Check sheet for the modelled part. Datum: model origin and axes. Units: mm. Face numbers are marked on the shaded views. A direction names the side the tool comes from. Give positions to 0.01 mm unless a question says otherwise; leave off trailing zeros. Loops run counter-clockwise (first coordinate to the right, second up) from the corner with the lowest first, then second, coordinate; pieces in that order, holes last. Notation, with made-up numbers: M 12,63.5 L 33,63.5 A19 ccw 33,93.5 Z; hole C 32.5,76 d7. An arc over 180 degrees is marked long. Put each result on its own line as item: value. Start each with the question number.
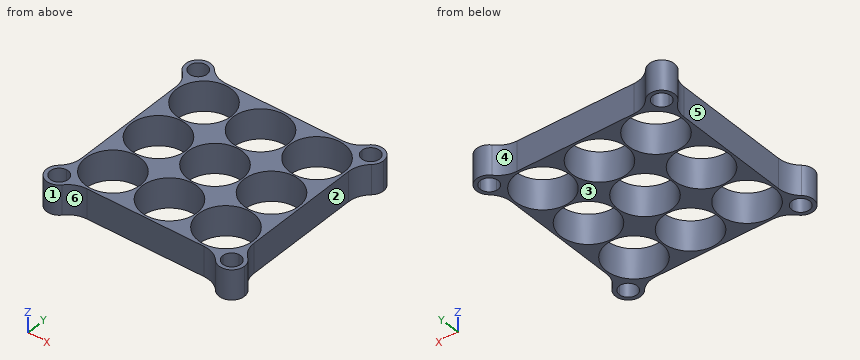
```python
from build123d import *

# Parameters (mm, degrees)
F0_R     = 9.25
F1_DEPTH = 10
F2_R     = 8


with BuildPart() as f1:
    # F0 (on Top) → F1 (new body)
    with BuildSketch(Plane.XY):
        with BuildLine():
            Line((22.3468586802, 59.2135186791), (-27.1531413198, 59.2135186791))
            ThreePointArc((-27.1531413198, 59.2135186791), (-28.3979374997, 56.2083148591), (-31.4031413198, 54.9635186791))
            Line((-31.4031413198, 54.9635186791), (-31.4031413198, 5.4635186791))
            ThreePointArc((-31.4031413198, 5.4635186791), (-28.3979374997, 4.2187224992), (-27.1531413198, 1.2135186791))
            Line((-27.1531413198, 1.2135186791), (22.3468586802, 1.2135186791))
            ThreePointArc((22.3468586802, 1.2135186791), (23.5916548602, 4.2187224992), (26.5968586802, 5.4635186791))
            Line((26.5968586802, 5.4635186791), (26.5968586802, 54.9635186791))
            ThreePointArc((26.5968586802, 54.9635186791), (23.5916548602, 56.2083148591), (22.3468586802, 59.2135186791))
        make_face()
        with Locations((-21.4031413198, 11.2135186791)):
            Circle(F0_R, mode=Mode.SUBTRACT)
        with Locations((-2.4031413198, 11.2135186791)):
            Circle(F0_R, mode=Mode.SUBTRACT)
        with Locations((16.5968586802, 11.2135186791)):
            Circle(F0_R, mode=Mode.SUBTRACT)
        with Locations((-21.4031413198, 30.2135186791)):
            Circle(F0_R, mode=Mode.SUBTRACT)
        with Locations((-21.4031413198, 49.2135186791)):
            Circle(F0_R, mode=Mode.SUBTRACT)
        with Locations((-2.4031413198, 30.2135186791)):
            Circle(F0_R, mode=Mode.SUBTRACT)
        with Locations((16.5968586802, 30.2135186791)):
            Circle(F0_R, mode=Mode.SUBTRACT)
        with Locations((-2.4031413198, 49.2135186791)):
            Circle(F0_R, mode=Mode.SUBTRACT)
        with Locations((16.5968586802, 49.2135186791)):
            Circle(F0_R, mode=Mode.SUBTRACT)
        with BuildLine():
            Line((-28.4031413198, 59.2135186791), (-27.1531413198, 59.2135186791))
            ThreePointArc((-27.1531413198, 59.2135186791), (-34.4083451398, 62.2187224992), (-31.4031413198, 54.9635186791))
            Line((-31.4031413198, 54.9635186791), (-31.4031413198, 56.2135186791))
            ThreePointArc((-31.4031413198, 56.2135186791), (-33.5244616633, 61.3348390227), (-28.4031413198, 59.2135186791))
        make_face()
        with BuildLine():
            ThreePointArc((-31.4031413198, 54.9635186791), (-28.3979374997, 56.2083148591), (-27.1531413198, 59.2135186791))
            Line((-27.1531413198, 59.2135186791), (-28.4031413198, 59.2135186791))
            ThreePointArc((-28.4031413198, 59.2135186791), (-29.2818209762, 57.0921983356), (-31.4031413198, 56.2135186791))
            Line((-31.4031413198, 56.2135186791), (-31.4031413198, 54.9635186791))
        make_face()
        with BuildLine():
            ThreePointArc((-27.1531413198, 1.2135186791), (-28.3979374997, 4.2187224992), (-31.4031413198, 5.4635186791))
            Line((-31.4031413198, 5.4635186791), (-31.4031413198, 4.2135186791))
            ThreePointArc((-31.4031413198, 4.2135186791), (-29.2818209762, 3.3348390227), (-28.4031413198, 1.2135186791))
            Line((-28.4031413198, 1.2135186791), (-27.1531413198, 1.2135186791))
        make_face()
        with BuildLine():
            Line((-31.4031413198, 4.2135186791), (-31.4031413198, 5.4635186791))
            ThreePointArc((-31.4031413198, 5.4635186791), (-34.4083451398, -1.7916851409), (-27.1531413198, 1.2135186791))
            Line((-27.1531413198, 1.2135186791), (-28.4031413198, 1.2135186791))
            ThreePointArc((-28.4031413198, 1.2135186791), (-33.5244616633, -0.9078016644), (-31.4031413198, 4.2135186791))
        make_face()
        with BuildLine():
            Line((26.5968586802, 4.2135186791), (26.5968586802, 5.4635186791))
            ThreePointArc((26.5968586802, 5.4635186791), (23.5916548602, 4.2187224992), (22.3468586802, 1.2135186791))
            Line((22.3468586802, 1.2135186791), (23.5968586802, 1.2135186791))
            ThreePointArc((23.5968586802, 1.2135186791), (24.4755383367, 3.3348390227), (26.5968586802, 4.2135186791))
        make_face()
        with BuildLine():
            ThreePointArc((30.8468586802, 1.2135186791), (29.6020625003, 4.2187224992), (26.5968586802, 5.4635186791))
            Line((26.5968586802, 5.4635186791), (26.5968586802, 4.2135186791))
            ThreePointArc((26.5968586802, 4.2135186791), (28.7181790238, 3.3348390227), (29.5968586802, 1.2135186791))
            ThreePointArc((29.5968586802, 1.2135186791), (26.5968586802, -1.7864813209), (23.5968586802, 1.2135186791))
            Line((23.5968586802, 1.2135186791), (22.3468586802, 1.2135186791))
            ThreePointArc((22.3468586802, 1.2135186791), (26.5968586802, -3.0364813209), (30.8468586802, 1.2135186791))
        make_face()
        with BuildLine():
            Line((23.5968586802, 59.2135186791), (22.3468586802, 59.2135186791))
            ThreePointArc((22.3468586802, 59.2135186791), (23.5916548602, 56.2083148591), (26.5968586802, 54.9635186791))
            Line((26.5968586802, 54.9635186791), (26.5968586802, 56.2135186791))
            ThreePointArc((26.5968586802, 56.2135186791), (24.4755383367, 57.0921983356), (23.5968586802, 59.2135186791))
        make_face()
        with BuildLine():
            ThreePointArc((30.8468586802, 59.2135186791), (26.5968586802, 63.4635186791), (22.3468586802, 59.2135186791))
            Line((22.3468586802, 59.2135186791), (23.5968586802, 59.2135186791))
            ThreePointArc((23.5968586802, 59.2135186791), (26.5968586802, 62.2135186791), (29.5968586802, 59.2135186791))
            ThreePointArc((29.5968586802, 59.2135186791), (28.7181790238, 57.0921983356), (26.5968586802, 56.2135186791))
            Line((26.5968586802, 56.2135186791), (26.5968586802, 54.9635186791))
            ThreePointArc((26.5968586802, 54.9635186791), (29.6020625003, 56.2083148591), (30.8468586802, 59.2135186791))
        make_face()
    extrude(amount=F1_DEPTH)

    # F2
    f2_edges = [f1.edges().sort_by_distance(p)[0] for p in [
        (26.596859, 54.963519, 5),
        (22.346859, 59.213519, 5),
        (-27.153141, 59.213519, 5),
        (-27.153141, 1.213519, 5),
        (-31.403141, 5.463519, 5),
        (-31.403141, 54.963519, 5),
        (22.346859, 1.213519, 5),
        (26.596859, 5.463519, 5),
    ]]
    fillet(f2_edges, radius=F2_R)


solid = f1.part
```
Q1. Access from +Z, -Z, +X, -X, +Y, -Y to the whole of each face (thin tool, end or side, straight path). Record for the marked faces 4, 5 and 6.
Q2. Section check C-C, the plane z = 5.75. Give the number of separate pieces and of enclosed holes in the cut face, then the cut area to 3 significant figures.
Q3. Mould release check, pull along X, two halves, no side actions. Record for the marked faces 1, 2 and 3: pulls with the +X half, pulls with the -X half, needs draft (parallel to the pull), parting line crosses it, or undercut.
Q4. Section check B-B, the plane y = 41.5. Record the cut outline in (x, z).
Q5. Section check A-A, the plane x = -27. Record the cut outline in (y, z), then the cut area to 3 significant figures.
Q6. Depth check by flat-ended pin: P1, Ø5, axis at y = 24, z = 3, coming from the -X side; P2, Ø10, axis at x = 22, y = 8.5, coming from the -Z side; P3, Ø2, axis at x = 8, z = 3, coming from the -Y side; P4, Ø1, axis at y = 35.5, z = 3.5, coming from the +X side. Enter the tip coordinate at first touch or a pass-through.
Q7. Thickness scan on line 1 along X through (y, z) = (14, 7.75); line 2 along X through (y, z) = (19.5, 4.75); line 3 along Y through (x, z) = (-10, 7.25). Record the ranges inside material, lowest first. Write a range as [from, to].
Found:
1. face 4: +Z, -Z, +Y
1. face 5: +Z, -Z, -X
1. face 6: +Z, -Z, -Y
2. separate pieces: 1
2. enclosed holes: 13
2. area: 1,030 mm^2
3. face 1: undercut
3. face 2: pulls with the +X half
3. face 3: needs draft
4. outline: M -31.4,0 L -26.51,0 L -26.51,10 L -31.4,10 Z; M -16.3,0 L -7.51,0 L -7.51,10 L -16.3,10 Z; M 2.7,0 L 11.49,0 L 11.49,10 L 2.7,10 Z; M 21.7,0 L 26.6,0 L 26.6,10 L 21.7,10 Z
5. outline: M -0.44,0 L 3.85,0 L 3.85,10 L -0.44,10 Z; M 18.58,0 L 22.85,0 L 22.85,10 L 18.58,10 Z; M 37.58,0 L 41.85,0 L 41.85,10 L 37.58,10 Z; M 56.58,0 L 60.87,0 L 60.87,10 L 56.58,10 Z
5. area: 171 mm^2
6. P1: stops at x = -31.4
6. P2: stops at z = 0
6. P3: stops at y = 1.21
6. P4: stops at x = 26.6
7. line 1: x = [-31.4, -30.22], [-12.58, -11.22], [6.42, 7.78], [25.42, 26.6]
7. line 2: x = [-31.4, -25.51], [-17.29, -6.51], [1.71, 12.49], [20.71, 26.6]
7. line 3: y = [1.21, 5.94], [16.49, 24.94], [35.49, 43.94], [54.49, 59.21]
